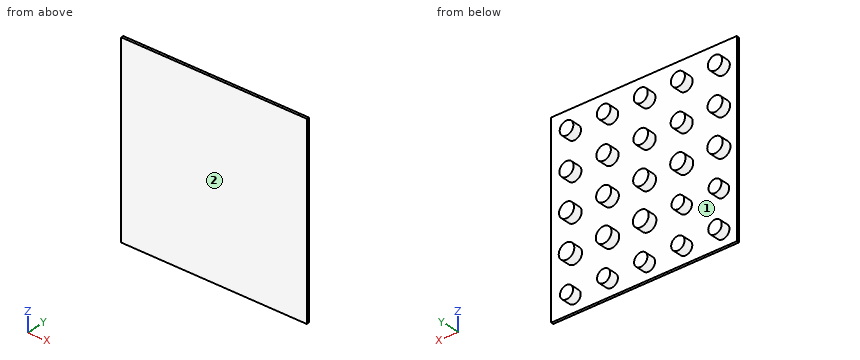
from build123d import *

# Parameters (mm, degrees)
SKETCH1_W           = 38.1
SKETCH1_H           = 38.1
BOSS_EXTRUDE1_DEPTH = 0.508
SKETCH2_R           = 1.3843
SKETCH2_R_2         = 1.3716
SKETCH2_R_3         = 1.3589
SKETCH2_R_4         = 1.3462
SKETCH2_R_5         = 1.3335
SKETCH2_R_6         = 1.3081
SKETCH2_R_7         = 1.6256
SKETCH2_R_8         = 1.6129
SKETCH2_R_9         = 1.6002
SKETCH2_R_10        = 1.5748
SKETCH2_R_11        = 1.5621
SKETCH2_R_12        = 1.5494
SKETCH2_R_13        = 1.5367
SKETCH2_R_14        = 1.4732
SKETCH2_R_15        = 1.4986
SKETCH2_R_16        = 1.4859
SKETCH2_R_17        = 1.4478
SKETCH2_R_18        = 1.4351
SKETCH2_R_19        = 1.4097
SKETCH2_R_20        = 1.397
SKETCH2_R_21        = 1.3208
SKETCH2_R_22        = 1.5875
SKETCH2_R_23        = 1.524
SKETCH2_R_24        = 1.4605
BOSS_EXTRUDE2_DEPTH = 1.905


with BuildPart() as part:
    # Sketch1 → Boss-Extrude1 (new body)
    with BuildSketch(Plane(origin=(0, 0, 0), x_dir=(1, 0, 0), z_dir=(0, 1, 0))):
        Rectangle(SKETCH1_W, SKETCH1_H)
    extrude(amount=BOSS_EXTRUDE1_DEPTH)

    # Sketch2 → Boss-Extrude2 (add)
    with BuildSketch(Plane(origin=(0, 0.508, 0), x_dir=(1, 0, 0), z_dir=(0, 1, 0))):
        with Locations((-16.163328468, 16.163328468)):
            Circle(SKETCH2_R)
        with Locations((-8.543328468, 16.163328468)):
            Circle(SKETCH2_R_2)
        with Locations((-0.923328468, 16.163328468)):
            Circle(SKETCH2_R_3)
        with Locations((6.696671532, 16.163328468)):
            Circle(SKETCH2_R_4)
        with Locations((14.316671532, 16.163328468)):
            Circle(SKETCH2_R_5)
        with Locations((-8.543328468, 8.543328468)):
            Circle(SKETCH2_R_6)
        with Locations((-0.923328468, 8.543328468)):
            Circle(SKETCH2_R_7)
        with Locations((6.696671532, 8.543328468)):
            Circle(SKETCH2_R_8)
        with Locations((14.316671532, 8.543328468)):
            Circle(SKETCH2_R_9)
        with Locations((-8.543328468, 0.923328468)):
            Circle(SKETCH2_R_10)
        with Locations((-0.923328468, 0.923328468)):
            Circle(SKETCH2_R_11)
        with Locations((6.696671532, 0.923328468)):
            Circle(SKETCH2_R_12)
        with Locations((14.316671532, 0.923328468)):
            Circle(SKETCH2_R_13)
        with Locations((-8.543328468, -6.696671532)):
            Circle(SKETCH2_R_14)
        with Locations((-0.923328468, -6.696671532)):
            Circle(SKETCH2_R_15)
        with Locations((6.696671532, -6.696671532)):
            Circle(SKETCH2_R_16)
        with Locations((14.316671532, -6.696671532)):
            Circle(SKETCH2_R_14)
        with Locations((-8.543328468, -14.316671532)):
            Circle(SKETCH2_R_17)
        with Locations((-0.923328468, -14.316671532)):
            Circle(SKETCH2_R_18)
        with Locations((6.696671532, -14.316671532)):
            Circle(SKETCH2_R_19)
        with Locations((14.316671532, -14.316671532)):
            Circle(SKETCH2_R_20)
        with Locations((-16.163328468, 8.543328468)):
            Circle(SKETCH2_R_21)
        with Locations((-16.163328468, 0.923328468)):
            Circle(SKETCH2_R_22)
        with Locations((-16.163328468, -6.696671532)):
            Circle(SKETCH2_R_23)
        with Locations((-16.163328468, -14.316671532)):
            Circle(SKETCH2_R_24)
    extrude(amount=BOSS_EXTRUDE2_DEPTH)


solid = part.part
Could you check a few things on this model? Use its own coordinates, in mm. Face numbers are marked on the shaded views. Give positions to 0.01 mm unless a question says otherwise; leave off trailing zeros. Order: outer loops, then holes, each group sorted by start corner. A loop starts at its lowest first (then second) coordinate and runs counter-clockwise, first axis right, second up.
Item 1: If we mould it in two halves opening along X, with no side actions, what happens to the marked faces 1 and 2? For each: pulls with the +X half, pulls with the -X half, needs draft (parallel to the pull), parting line crosses it, or undercut.
Item 2: If we section it at B-B, the plane z = -8: Write out the boundary of the cut face in (x, y).
Item 3: If we section it at D-D, the plane z = 11: Write out the boundary of the cut face in (x, y), plus the area to 3 significant figures.
Item 4: If we section it at C-C, the plane x = 0: Write out the boundary of the cut face in (y, z).
Item 5: I need wall thicknesses on line 1 (Z direction, x = -16, y = 1.8); line 2 (X direction, y = 1.4, z = -8); line 3 (X direction, y = 0.6, z = 15). Which ranges of each line are inside material? Lowest first, please.
Item 6: I'm going to push flat-ended pins straight in: pin 1 (3 mm diameter, centred on x = 4.5, z = 9, fed in from +Y); pin 2 (1 mm diameter, centred on x = -12, z = 10, fed in from -Y). Where does each tip first touch, or does it pass through?
Item 7: If we section it at A-A, the plane y = 1.35: Count the separate pieces of the cut face and the enclosed holes in it, plus the area to 3 significant figures.
Values:
1. face 1: undercut
1. face 2: needs draft
2. outline: (-19.05, 0) - (19.05, 0) - (19.05, 0.51) - (15.82, 0.51) - (15.82, 2.41) - (12.81, 2.41) - (12.81, 0.51) - (8.22, 0.51) - (8.22, 2.41) - (5.18, 2.41) - (5.18, 0.51) - (0.61, 0.51) - (0.61, 2.41) - (-2.46, 2.41) - (-2.46, 0.51) - (-7.35, 0.51) - (-7.35, 2.41) - (-9.73, 2.41) - (-9.73, 0.51) - (-14.96, 0.51) - (-14.96, 2.41) - (-17.37, 2.41) - (-17.37, 0.51) - (-19.05, 0.51) - close
3. outline: (-19.05, 0) - (19.05, 0) - (19.05, 0.51) - (-19.05, 0.51) - close
3. area: 19.4 mm2
4. outline: (0, -19.05) - (0.51, -19.05) - (0.51, -17.16) - (2.41, -17.16) - (2.41, -15.17) - (0.51, -15.17) - (0.51, -9.88) - (2.41, -9.88) - (2.41, -7.21) - (0.51, -7.21) - (0.51, -2.18) - (2.41, -2.18) - (2.41, 0.34) - (0.51, 0.34) - (0.51, 5.52) - (2.41, 5.52) - (2.41, 7.88) - (0.51, 7.88) - (0.51, 13.22) - (2.41, 13.22) - (2.41, 15.42) - (0.51, 15.42) - (0.51, 19.05) - (0, 19.05) - close
5. line 1: z = -17.54 to -14.79, -9.85 to -7.23, -2.5 to 0.66, 5.18 to 8.21, 12.87 to 15.77
5. line 2: x = -17.37 to -14.96, -9.73 to -7.35, -2.46 to 0.61, 5.18 to 8.22, 12.81 to 15.82
5. line 3: x = -17.45 to -14.87, -9.82 to -7.27, -2.19 to 0.34, 5.46 to 7.93, 13.1 to 15.54
6. pin 1: stops at y = 0.51
6. pin 2: stops at y = 0
7. separate pieces: 25
7. enclosed holes: 0
7. area: 170 mm2
